```python
from build123d import *


with BuildPart() as f1:
    # F0 (on Front) → F1 (revolve)
    with BuildSketch(Plane.XZ):
        with BuildLine():
            Line((45, 22.972104), (25.5, 22.972104))
            Line((25.5, 22.972104), (25.5, 17.872104))
            Line((25.5, 17.872104), (28.206175, 17.872104))
            ThreePointArc((28.206175, 17.872104), (29.872886, 17.366513), (30.977813, 16.020154))
            Line((30.977813, 16.020154), (31.899439, 13.795154))
            ThreePointArc((31.899439, 13.795154), (32.1278, 12.647104), (31.899439, 11.499054))
            Line((31.899439, 11.499054), (30.686249, 8.570154))
            ThreePointArc((30.686249, 8.570154), (30.457887, 7.422104), (30.686249, 6.274054))
            Line((30.686249, 6.274054), (31.899439, 3.345154))
            ThreePointArc((31.899439, 3.345154), (32.1278, 2.197104), (31.899439, 1.049054))
            Line((31.899439, 1.049054), (30.977813, -1.175946))
            ThreePointArc((30.977813, -1.175946), (29.872886, -2.522305), (28.206175, -3.027896))
            Line((28.206175, -3.027896), (27.959198, -3.027896))
            Line((27.959198, -3.027896), (25.5, -3.027896))
            Line((25.5, -3.027896), (25.5, -8.127896))
            Line((25.5, -8.127896), (45, -8.127896))
            Line((45, -8.127896), (45, 22.972104))
        make_face()
    revolve(axis=Axis((0, 0, 7.422104), (0, 0, -1)))


solid = f1.part
```
For this review, take the finished solid that the model builds, in its own axes (mm). A direction names the side the tool comes from. Give positions to 0.01 mm unless a question says otherwise; leave off trailing zeros.
1) Insertion check: pin 1 (1 mm diameter, centred on y = -30.5, z = -4.5, fed in from +X); pin 2 (1.5 mm diameter, centred on x = -8, z = -3.5, fed in from -Y); pin 3 (1 mm diameter, centred on y = 10, z = -3, fed in from +X). Each pin has a flat end and moves straight along its axis. Give the tip position at first contact, or say it passes through.
2) Wall thickness on line 1 (Z direction, x = 17, y = 27); line 2 (Y direction, x = 0, z = 19.55): over which ranges is each line inside the solid? List them lowest first.
3) The part is to be moulded in two halves that separate along Z. For faces 1 (the face through (-19, 19, -8.128)), 2 (the face through (-6.665, 30.014, 8.712)), 3 (the face through (19, 19, 22.972)), 4 (the face through (20.765, 39.923, 7.64)), say which applies: released by +Z, released by -Z, zero draft, split by the parting line, or undercut.
4) For faces 5 (the face through (6, 25, 17.872)), 6 (the face through (-5.5, 24.9, -5.6)), list the 3-axis set-ups (+Z, -Z, +X, -X, +Y, -Y) from which the entire face can be reached by the end or side of a thin tool; tool diameter is ignored.
Derived:
1. pin 1: stops at x = 33.54
1. pin 2: stops at y = -44.41
1. pin 3: stops at x = 43.99
2. line 1: z = -8.13 to 1.07, 3.33 to 11.52, 13.78 to 22.97
2. line 2: y = -45 to -25.5, 25.5 to 45
3. face 1: released by -Z
3. face 2: undercut
3. face 3: released by +Z
3. face 4: zero draft
4. face 5: none
4. face 6: +Z, -Z
